Autodesk Inventor part; units mm, degrees
ref_plane "YZ Plane" through (0, 0, 0) normal (1, 0, 0) x (0, 1, 0)
ref_plane "XZ Plane" through (0, 0, 0) normal (0, 1, 0) x (-1, 0, 0)
ref_plane "XY Plane" through (0, 0, 0) normal (0, 0, 1) x (1, 0, 0)
sketch "Sketch1" plane through (0, 0, 0) normal (0, 1, 0) x (-1, 0, 0)
  circle A0 centre (-20.8, 14.4) radius 13.125
  circle A1 centre (-42.7, -7.5) radius 1.875
  circle A2 centre (1.1, 36.3) radius 1.875
  circle A3 centre (1.1, -7.5) radius 1.875
  circle A4 centre (-42.7, 36.3) radius 1.875
  circle A5 centre (-6.4, 35.2) radius 2.0734
  circle A6 centre (-35.2, -6.4) radius 2.0734
  circle A7 centre (-6.4, -6.4) radius 2.0734
  circle A8 centre (0, 0) radius 2.0734
  line L0 (-37.85, 31.45) -> (-37.85, -2.65)
  line L1 (-3.75, 31.45) -> (-37.85, 31.45)
  line L2 (-3.75, -2.65) -> (-3.75, 31.45)
  line L3 (-37.85, -2.65) -> (-3.75, -2.65)
  circle A9 centre (0, 28.8) radius 2.0734
  circle A10 centre (-35.2, 35.2) radius 2.0734
  circle A11 centre (-41.6, 0) radius 2.0734
  circle A12 centre (-41.6, 28.8) radius 2.0734
  line L4 (-43.7, 39.275) -> (2.1, 39.275)
  arc A13 (-43.7, 39.275) -> (-45.675, 37.3) centre (-43.7, 37.3) ccw
  line L5 (-45.675, -8.5) -> (-45.675, 37.3)
  arc A14 (-45.675, -8.5) -> (-43.7, -10.475) centre (-43.7, -8.5) ccw
  line L6 (2.1, -10.475) -> (-43.7, -10.475)
  arc A15 (2.1, -10.475) -> (4.075, -8.5) centre (2.1, -8.5) ccw
  line L7 (4.075, 37.3) -> (4.075, -8.5)
  arc A16 (4.075, 37.3) -> (2.1, 39.275) centre (2.1, 37.3) ccw
  line L8 (-3.75, 14.4) -> (-37.85, 14.4)
  dimension "d36" = 26.25
extrude "Extrusion1" add sketch "Sketch1" along normal blind 3.75 contours L8 L2 L3 L0 A0 | A0 L8 L0 L1 L2 | A1 | A2 | A3 | A4 | L4 A16 L7 A15 L6 A14 L5 A13
properties part number "Camera Mount Top"
The model under review builds one solid part; all positions refer to its coordinate system, in mm. Give positions to 0.01 mm unless a question says otherwise; leave off trailing zeros. Write each loop counter-clockwise with the first axis right and the second up, starting at its lowest first coordinate (ties: lowest second). Pieces come first, ordered by that corner, then holes. Notation, with made-up numbers: (73.5, -2.5) -> (89.5, -2.5) arc R23 cw to (89.5, 31.5) -> close; hole circle Ø6 at (48, 10.25). An arc over 180 degrees is marked (long way). Answer in a Markdown table with one row per item.
1) Mouldability with a two-part tool opening along Z and no side actions: class faces 1 (the cylindrical face through (1.645, 1.849, 1.262)), 2 (the flat face through (32, 3.75, 26)), 3 (the cylindrical face through (36.845, 1.849, 36.462)), 4 (the flat face through (20, 2, -10.475)) as +Z half, -Z half, draft (parallel to the pull), parting line (faces both ways), or undercut.
Worked answers:
| item | result |
|---|---|
| face 1 | undercut |
| face 2 | draft |
| face 3 | undercut |
| face 4 | -Z half |
2) Clearance check with a flat-ended pin moving along its axis: P1, Ø2.5, axis at x = 35.2, z = 35.2, coming from the +Y side. State where the tip first meets the part, or that it passes through.
Worked answers:
| item | result |
|---|---|
| P1 | through |
3) Add section A-A on z = -6.4. State the section outline as (x, y) points (3 decimals), plus the area to 3 significant figures.
Worked answers:
| item | result |
|---|---|
| outline | (-4.075, 0) -> (4.327, 0) -> (4.327, 3.75) -> (-4.075, 3.75) -> close; (8.473, 0) -> (33.127, 0) -> (33.127, 3.75) -> (8.473, 3.75) -> close; (37.273, 0) -> (45.675, 0) -> (45.675, 3.75) -> (37.273, 3.75) -> close |
| area | 155 mm² |
4) Add section D-D on y = 1.8. Count the separate pieces of the cut face and the enclosed holes in it, plus the area to 3 significant figures.
Worked answers:
| item | result |
|---|---|
| separate pieces | 1 |
| enclosed holes | 9 |
| area | 1,820 mm² |
5) Add section C-C on x = 20.8. State the section outline as (y, z) points (3 decimals).
Worked answers:
| item | result |
|---|---|
| outline | (0, -10.475) -> (3.75, -10.475) -> (3.75, 1.275) -> (0, 1.275) -> close; (0, 27.525) -> (3.75, 27.525) -> (3.75, 39.275) -> (0, 39.275) -> close |
6) Add section B-B on x = 41.6. State the section outline as (y, z) points (3 decimals), plus the area to 3 significant figures.
Worked answers:
| item | result |
|---|---|
| outline | (0, -10.475) -> (3.75, -10.475) -> (3.75, -2.073) -> (0, -2.073) -> close; (0, 2.073) -> (3.75, 2.073) -> (3.75, 26.727) -> (0, 26.727) -> close; (0, 30.873) -> (3.75, 30.873) -> (3.75, 39.275) -> (0, 39.275) -> close |
| area | 155 mm² |
7) For L1, parallel to Z at x = 0, y = 1.7 (3 decimals); L2, parallel to Z at x = 6.4, y = 0.95 (3 decimals); L3, parallel to X at y = 1.4, z = 23 (3 decimals), list the stretches that pass through material, from the lowest coordinate up. Write a range as [from, to].
Worked answers:
| item | result |
|---|---|
| L1 | [-10.475, -2.073], [2.073, 26.727], [30.873, 39.275] |
| L2 | [-10.475, -8.473], [-4.327, 33.127], [37.273, 39.275] |
| L3 | [-4.075, 10.885], [30.715, 45.675] |
